from build123d import *

# Parameters (mm, degrees)
SKETCH1_R           = 17.399
BOSS_EXTRUDE1_DEPTH = 23.0000048
SKETCH2_R           = 2.5
BOSS_EXTRUDE2_DEPTH = 10
SKETCH3_R           = 1.499997
BOSS_EXTRUDE3_DEPTH = 2
SKETCH4_R           = 1.524
SKETCH4_R_2         = 1.5
CUT_EXTRUDE1_DEPTH  = 2


with BuildPart() as part:
    # Sketch1 → Boss-Extrude1 (new body)
    with BuildSketch(Plane(origin=(0, 0, 0), x_dir=(1, 0, 0), z_dir=(0, 1, 0))):
        with Locations(Location((0, 0, 0), (0, 0, 270))):
            Circle(SKETCH1_R)
    extrude(amount=BOSS_EXTRUDE1_DEPTH)

    # Sketch2 → Boss-Extrude2 (add)
    with BuildSketch(Plane(origin=(0, 23.0000048, 0), x_dir=(1, 0, 0), z_dir=(0, 1, 0))):
        with Locations(Location((0, 0, 0), (0, 0, 270))):
            Circle(SKETCH2_R)
    extrude(amount=BOSS_EXTRUDE2_DEPTH)

    # Sketch3 → Boss-Extrude3 (add)
    with BuildSketch(Plane.XZ):
        with Locations(Location((0, 0, 0), (0, 0, 90))):
            Circle(SKETCH3_R)
    extrude(amount=BOSS_EXTRUDE3_DEPTH)

    # Sketch4 → Cut-Extrude1 (cut)
    with BuildSketch(Plane.XZ):
        with Locations(Location((0, 12.5000004, 0), (0, 0, 270))):
            Circle(SKETCH4_R)
        with Locations(Location((9.4999937, 0, 0), (0, 0, 270))):
            Circle(SKETCH4_R_2)
        with Locations(Location((-9.4999937, 0, 0), (0, 0, 90))):
            Circle(SKETCH4_R_2)
        with Locations(Location((0, -12.5000004, 0), (0, 0, 90))):
            Circle(SKETCH4_R)
    extrude(amount=-CUT_EXTRUDE1_DEPTH, mode=Mode.SUBTRACT)


solid = part.part
CAD build for the part. Positions are in the model's coordinates, mm. A direction names the side the tool comes from. Round coordinates to 2 decimals unless told otherwise and drop trailing zeros. Write each loop counter-clockwise with the first axis right and the second up, starting at its lowest first coordinate (ties: lowest second). Pieces come first, ordered by that corner, then holes. Notation, with made-up numbers: M -30.75,-0.75 L 6.25,-0.75 A27 cw 6.25,16.25 Z; hole C 83,23 d11. An arc over 180 degrees is marked long. Use a Markdown table: item, result. Add a question column.
1. Slice it at D-D on y = 29. Give the cut face in (x, z).
2. Slice it at C-C on x = 0. Give the cut face in (y, z), then the cut area to 3 significant figures.
3. Slice it at A-A on y = 1.5. Give the cut face in (x, z), then the cut area to 3 significant figures.
4. 3-axis set-ups, long thin cutter, end or side, ignore diameter. For faces 1 (the face through (0, 2, -13)), 2 (the face through (0, -2, 0)), 3 (the face through (-2.44, 27.93, -0.54)): which of +Z, -Z, +X, -X, +Y, -Y reach the whole face in a straight line?
5. Drill centre lines: probe 1 along Y at (x, z) = (4.5, -8.5); probe 2 along X at (y, z) = (1.5, -12.5); probe 3 along X at (y, z) = (19, -4.5). Where is each one in solid material? Low to high.
6. Slice it at B-B on z = 0. Give the cut face in (x, y).
7. Flat gauge pins, fed straight in: P1, Ø10, axis at x = 5.5, y = 26, coming from the -Z side; P2, Ø10, axis at x = 0.5, z = -10.5, coming from the -Y side; P3, Ø1.8, axis at x = -9.5, z = 0, coming from the +Y side; P4, Ø12, axis at x = -5.5, y = 17.5, coming from the +Z side. Where does each tip first touch, or does it go through?
8. Pull direction Z, two halves, no side cores. Call faces 4 (the face through (-1.487, -0.986, -0.195)), 5 (the face through (0, 33, 0)), 6 (the face through (0, 2, 13)), 7 (the face through (10, 2, 0)): released by +Z, released by -Z, zero draft, split by the parting line, or undercut.
Reply:
| question | item | result |
|---|---|---|
| 1 | outline | C 0,0 d5 |
| 2 | outline | M -2,-1.5 L 0,-1.5 L 0,-10.98 L 2,-10.98 L 2,-14.02 L 0,-14.02 L 0,-17.4 L 23,-17.4 L 23,-2.5 L 33,-2.5 L 33,2.5 L 23,2.5 L 23,17.4 L 0,17.4 L 0,14.02 L 2,14.02 L 2,10.98 L 0,10.98 L 0,1.5 L -2,1.5 Z |
| 2 | area | 844 mm^2 |
| 3 | outline | C 0,0 d34.8; hole C -9.5,0 d3; hole C 0,-12.5 d3.05; hole C 0,12.5 d3.05; hole C 9.5,0 d3 |
| 3 | area | 922 mm^2 |
| 4 | face 1 | -Y |
| 4 | face 2 | +Z, -Z, +X, -X, -Y |
| 4 | face 3 | +Y |
| 5 | probe 1 | y = 0 to 23 |
| 5 | probe 2 | x = -12.1 to -1.52, 1.52 to 12.1 |
| 5 | probe 3 | x = -16.81 to 16.81 |
| 6 | outline | M -17.4,0 L -11,0 L -11,2 L -8,2 L -8,0 L -1.5,0 L -1.5,-2 L 1.5,-2 L 1.5,0 L 8,0 L 8,2 L 11,2 L 11,0 L 17.4,0 L 17.4,23 L 2.5,23 L 2.5,33 L -2.5,33 L -2.5,23 L -17.4,23 Z |
| 7 | P1 | stops at z = -17.33 |
| 7 | P2 | stops at y = 0 |
| 7 | P3 | stops at y = 23 |
| 7 | P4 | stops at z = 17.4 |
| 8 | face 4 | split by the parting line |
| 8 | face 5 | zero draft |
| 8 | face 6 | undercut |
| 8 | face 7 | undercut |
